from build123d import *

# Parameters (mm, degrees)
SKETCH1_R           = 6.5
BOSS_EXTRUDE1_DEPTH = 38.1
SKETCH2_R           = 19.05
BOSS_EXTRUDE2_DEPTH = 1.27
SKETCH3_R           = 1.2
CUT_EXTRUDE1_DEPTH  = 48.705365526
SKETCH4_R           = 1.75
CUT_EXTRUDE2_DEPTH  = 7.62


with BuildPart() as part:
    # Sketch1 → Boss-Extrude1 (new body)
    with BuildSketch(Plane.XY):
        with Locations(Location((0, 0, 0), (0, 0, 180))):
            Circle(SKETCH1_R)
    extrude(amount=BOSS_EXTRUDE1_DEPTH)

    # Sketch2 → Boss-Extrude2 (add)
    with BuildSketch(Plane.XY.offset(38.1)):
        Circle(SKETCH2_R)
    extrude(amount=BOSS_EXTRUDE2_DEPTH)

    # Sketch3 → Cut-Extrude1 (cut, through all)
    with BuildSketch(Plane(origin=(0, 0, 0), x_dir=(-1, 0, 0), z_dir=(0, 0, -1))):
        Circle(SKETCH3_R)
    extrude(amount=-CUT_EXTRUDE1_DEPTH, mode=Mode.SUBTRACT)

    # Sketch4 → Cut-Extrude2 (cut)
    with BuildSketch(Plane(origin=(0, 0, 38.1), x_dir=(-1, 0, 0), z_dir=(0, 0, -1))):
        with Locations((0, 9.398)):
            Circle(SKETCH4_R)
    extrude(amount=-CUT_EXTRUDE2_DEPTH, mode=Mode.SUBTRACT)


solid = part.part
Source: CAD feature listing. Evaluate the final solid. Frame: model axes, mm. A direction names the side the tool comes from. Coordinates: 2 decimals unless noted, no trailing zeros. Order: outer loops, then holes, each group sorted by start corner. A loop starts at its lowest first (then second) coordinate and runs counter-clockwise, first axis right, second up.
Item 1: Cut plane A-A (x = 0). Return loops of the section in (y, z).
Output values:
outline: (-19.05, 38.1) - (-6.5, 38.1) - (-6.5, 0) - (-1.2, 0) - (-1.2, 39.37) - (-19.05, 39.37) - close; (1.2, 0) - (6.5, 0) - (6.5, 38.1) - (7.65, 38.1) - (7.65, 39.37) - (1.2, 39.37) - close; (11.15, 38.1) - (19.05, 38.1) - (19.05, 39.37) - (11.15, 39.37) - close
Item 2: Set-up query: faces 1 (the face through (0, -4, 39.37)), 2 (the face through (5.158, 3.955, 18.783)). Return all of +Z, -Z, +X, -X, +Y, -Y with unobstructed straight access to the full face (end or side cutting, diameter ignored); none if empty.
Output values:
face 1: +Z, +X, -X, +Y, -Y
face 2: -Z
Item 3: First-contact query: P1, Ø5, axis at x = 3.5, y = -8.5, coming from the -Z side; P2, Ø12, axis at y = -4, z = 25.5, coming from the +X side; P3, Ø4, axis at x = -6.5, z = 34, coming from the +Y side. Flat tips, straight axial feed; report the tip coordinate or a pass-through.
Output values:
P1: stops at z = 38.1
P2: stops at x = 6.5
P3: stops at y = 4.69
Item 4: Cut plane D-D (y = -4.5). Return loops of the section in (x, z), plus the area to 3 significant figures.
Output values:
outline: (-18.51, 38.1) - (-4.69, 38.1) - (-4.69, 0) - (4.69, 0) - (4.69, 38.1) - (18.51, 38.1) - (18.51, 39.37) - (-18.51, 39.37) - close
area: 404 mm2
Item 5: Cut plane B-B (y = 0). Return loops of the section in (x, z).
Output values:
outline: (-19.05, 38.1) - (-6.5, 38.1) - (-6.5, 0) - (-1.2, 0) - (-1.2, 39.37) - (-19.05, 39.37) - close; (1.2, 0) - (6.5, 0) - (6.5, 38.1) - (19.05, 38.1) - (19.05, 39.37) - (1.2, 39.37) - close
Item 6: Cut plane C-C (z = 7). Return loops of the section in (x, y), plus the area to 3 significant figures.
Output values:
outline: circle Ø13 at (0, 0); hole circle Ø2.4 at (0, 0)
area: 128 mm2
Item 7: Material intervals for line 1 (Y direction, x = 0, z = 30); line 2 (Y direction, x = 0, z = 38.7); line 3 (Z direction, x = -15.5, y = 9.5), sorted ascending.
Output values:
line 1: y = -6.5 to -1.2, 1.2 to 6.5
line 2: y = -19.05 to -1.2, 1.2 to 7.65, 11.15 to 19.05
line 3: z = 38.1 to 39.37
